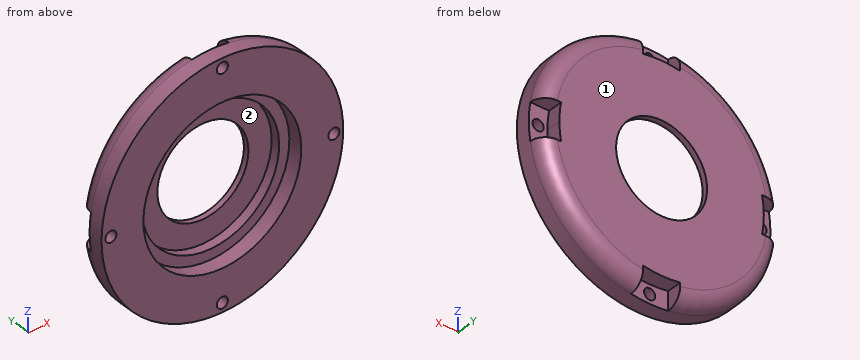
from build123d import *
from build123d.topology import SkipClean

# Parameters (mm, degrees)
SKETCH1_R           = 32.5
SKETCH1_R_2         = 27.5
BOSS_EXTRUDE1_DEPTH = 4
BOSS_EXTRUDE2_DEPTH = 4
SKETCH3_R           = 1.5
CUT_EXTRUDE1_DEPTH  = 6
BOSS_EXTRUDE4_START = -8
SKETCH7_R           = 25
BOSS_EXTRUDE4_DEPTH = 8
SKETCH8_R           = 27.5
SKETCH8_R_2         = 12.25
BOSS_EXTRUDE5_DEPTH = 4
SKETCH10_R          = 25
SKETCH10_R_2        = 12.25
BOSS_EXTRUDE6_DEPTH = 4
FILLET3_R           = 4
SKETCH11_R          = 21.25
CUT_EXTRUDE2_DEPTH  = 4
SKETCH14_R          = 18.5
CUT_EXTRUDE3_DEPTH  = 2.5


with BuildPart() as part:
    # Sketch1 → Boss-Extrude1 (new body)
    with BuildSketch(Plane(origin=(0, 0, 0), x_dir=(1, 0, 0), z_dir=(0, 1, 0))):
        with Locations(Location((0, 0, 0), (0, 0, 270))):
            Circle(SKETCH1_R)
        with Locations(Location((0, 0, 0), (0, 0, 270))):
            Circle(SKETCH1_R_2, mode=Mode.SUBTRACT)
    extrude(amount=BOSS_EXTRUDE1_DEPTH)

    # Sketch2 → Boss-Extrude2 (add)
    with SkipClean():  # the faces are left unmerged after this step: merging them gives an invalid solid
        with BuildSketch(Plane(origin=(0, 4, 0), x_dir=(1, 0, 0), z_dir=(0, 1, 0))):
            with BuildLine():
                ThreePointArc((-5, 32.113081447), (-22.980970389, 22.980970389), (-32.113081447, 5))
                Line((-32.113081447, 5), (-30, 5))
                Line((-30, 5), (-27.041634566, 5))
                ThreePointArc((-27.041634566, 5), (-19.445436483, 19.445436483), (-5, 27.041634566))
                Line((-5, 27.041634566), (-5, 32.113081447))
            make_face()
            with BuildLine():
                Line((-27.041634566, -5), (-32.113081447, -5))
                ThreePointArc((-32.113081447, -5), (-22.980970389, -22.980970389), (-5, -32.113081447))
                Line((-5, -32.113081447), (-5, -27.041634566))
                ThreePointArc((-5, -27.041634566), (-19.445436483, -19.445436483), (-27.041634566, -5))
            make_face()
            with BuildLine():
                Line((5, -27.041634566), (5, -32.113081447))
                ThreePointArc((5, -32.113081447), (22.980970389, -22.980970389), (32.113081447, -5))
                Line((32.113081447, -5), (27.041634566, -5))
                ThreePointArc((27.041634566, -5), (19.445436483, -19.445436483), (5, -27.041634566))
            make_face()
            with BuildLine():
                ThreePointArc((32.113081447, 5), (22.980970389, 22.980970389), (5, 32.113081447))
                Line((5, 32.113081447), (5, 27.041634566))
                ThreePointArc((5, 27.041634566), (19.445436483, 19.445436483), (27.041634566, 5))
                Line((27.041634566, 5), (32.113081447, 5))
            make_face()
        extrude(amount=BOSS_EXTRUDE2_DEPTH)

    # Sketch3 → Cut-Extrude1 (cut)
    with SkipClean():  # the faces are left unmerged after this step: merging them gives an invalid solid
        with BuildSketch(Plane(origin=(0, 4, 0), x_dir=(1, 0, 0), z_dir=(0, 1, 0))):
            with Locations(Location((0, 30, 0), (0, 0, 270))):
                Circle(SKETCH3_R)
            with Locations(Location((30, 0, 0), (0, 0, 270))):
                Circle(SKETCH3_R)
            with Locations(Location((0, -30, 0), (0, 0, 270))):
                Circle(SKETCH3_R)
            with Locations(Location((-30, 0, 0), (0, 0, 270))):
                Circle(SKETCH3_R)
        extrude(amount=-CUT_EXTRUDE1_DEPTH, mode=Mode.SUBTRACT)

    # Sketch7 → Boss-Extrude4 (add)
    # profile 1 of 5: a face of its own
    with BuildSketch(Plane(origin=(0, 8, 0), x_dir=(1, 0, 0), z_dir=(0, 1, 0)).offset(BOSS_EXTRUDE4_START)):
        with BuildLine():
            ThreePointArc((-27.041634566, 5), (-19.445436483, 19.445436483), (-5, 27.041634566))
            Line((-5, 27.041634566), (-5, 32.113081447))
            ThreePointArc((-5, 32.113081447), (-22.980970389, 22.980970389), (-32.113081447, 5))
            Line((-32.113081447, 5), (-27.041634566, 5))
        make_face()
    # profile 2 of 5: a face of its own
    with BuildSketch(Plane(origin=(0, 8, 0), x_dir=(1, 0, 0), z_dir=(0, 1, 0)).offset(BOSS_EXTRUDE4_START)):
        with BuildLine():
            Line((27.041634566, 5), (32.113081447, 5))
            ThreePointArc((32.113081447, 5), (22.980970389, 22.980970389), (5, 32.113081447))
            Line((5, 32.113081447), (5, 27.041634566))
            ThreePointArc((5, 27.041634566), (19.445436483, 19.445436483), (27.041634566, 5))
        make_face()
    # profile 3 of 5: a face of its own
    with BuildSketch(Plane(origin=(0, 8, 0), x_dir=(1, 0, 0), z_dir=(0, 1, 0)).offset(BOSS_EXTRUDE4_START)):
        with BuildLine():
            Line((5, -27.041634566), (5, -32.113081447))
            ThreePointArc((5, -32.113081447), (22.980970389, -22.980970389), (32.113081447, -5))
            Line((32.113081447, -5), (27.041634566, -5))
            ThreePointArc((27.041634566, -5), (19.445436483, -19.445436483), (5, -27.041634566))
        make_face()
    # profile 4 of 5: a face of its own
    with BuildSketch(Plane(origin=(0, 8, 0), x_dir=(1, 0, 0), z_dir=(0, 1, 0)).offset(BOSS_EXTRUDE4_START)):
        with BuildLine():
            Line((-27.041634566, -5), (-32.113081447, -5))
            ThreePointArc((-32.113081447, -5), (-22.980970389, -22.980970389), (-5, -32.113081447))
            Line((-5, -32.113081447), (-5, -27.041634566))
            ThreePointArc((-5, -27.041634566), (-19.445436483, -19.445436483), (-27.041634566, -5))
        make_face()
    # profile 5 of 5: a face of its own
    with BuildSketch(Plane(origin=(0, 8, 0), x_dir=(1, 0, 0), z_dir=(0, 1, 0)).offset(BOSS_EXTRUDE4_START)):
        with BuildLine():
            ThreePointArc((-27.041634566, -5), (-19.445436483, -19.445436483), (-5, -27.041634566))
            ThreePointArc((-5, -27.041634566), (0, -27.5), (5, -27.041634566))
            ThreePointArc((5, -27.041634566), (19.445436483, -19.445436483), (27.041634566, -5))
            ThreePointArc((27.041634566, -5), (27.385168893, -2.510482965), (27.5, 0))
            ThreePointArc((27.5, 0), (27.385168893, 2.510482965), (27.041634566, 5))
            ThreePointArc((27.041634566, 5), (19.445436483, 19.445436483), (5, 27.041634566))
            ThreePointArc((5, 27.041634566), (0, 27.5), (-5, 27.041634566))
            ThreePointArc((-5, 27.041634566), (-19.445436483, 19.445436483), (-27.041634566, 5))
            ThreePointArc((-27.041634566, 5), (-27.5, 0), (-27.041634566, -5))
        make_face()
        with Locations(Location((0, 0, 0), (0, 0, 270))):
            Circle(SKETCH7_R, mode=Mode.SUBTRACT)
    extrude(amount=BOSS_EXTRUDE4_DEPTH)

    # Sketch8 → Boss-Extrude5 (add)
    with BuildSketch(Plane(origin=(0, 0, 0), x_dir=(-1, 0, 0), z_dir=(0, -1, 0))):
        Circle(SKETCH8_R)
        with Locations(Location((0, 0, 0), (0, 0, 90))):
            Circle(SKETCH8_R_2, mode=Mode.SUBTRACT)
    extrude(amount=-BOSS_EXTRUDE5_DEPTH)

    # Sketch10 → Boss-Extrude6 (add)
    with BuildSketch(Plane(origin=(0, 4, 0), x_dir=(1, 0, 0), z_dir=(0, 1, 0))):
        Circle(SKETCH10_R)
        with Locations(Location((0, 0, 0), (0, 0, 90))):
            Circle(SKETCH10_R_2, mode=Mode.SUBTRACT)
    extrude(amount=BOSS_EXTRUDE6_DEPTH)

    # Fillet3
    fillet3_edges = [part.edges().sort_by_distance(p)[0] for p in [
        (22.980970389, 8, -22.980970389),
        (22.980970389, 8, 22.980970389),
        (-22.980970389, 8, 22.980970389),
        (-22.980970389, 8, -22.980970389),
    ]]
    fillet(fillet3_edges, radius=FILLET3_R - 0.0001)  # a hair under: the kernel refuses the full size

    # Sketch11 → Cut-Extrude2 (cut)
    with BuildSketch(Plane.XZ):
        with Locations(Location((0, 0, 0), (0, 0, 270))):
            Circle(SKETCH11_R)
    extrude(amount=-CUT_EXTRUDE2_DEPTH, mode=Mode.SUBTRACT)

    # Sketch14 → Cut-Extrude3 (cut)
    with BuildSketch(Plane.XZ.offset(-4)):
        with Locations(Location((0, 0, 0), (0, 0, 270))):
            Circle(SKETCH14_R)
    extrude(amount=-CUT_EXTRUDE3_DEPTH, mode=Mode.SUBTRACT)


solid = part.part
Input: part model. Units: mm. Frame: model coordinates. Face numbers are marked on the shaded views. Coordinates: 2 decimals unless noted, no trailing zeros. Loops run counter-clockwise (first coordinate to the right, second up) from the corner with the lowest first, then second, coordinate; pieces in that order, holes last.
(1) Material intervals for probe 1 along X at (y, z) = (3.2, 0); probe 2 along X at (y, z) = (1.1, -30); probe 3 along Z at (x, y) = (7, 3.75), sorted ascending.
(2) Pull-direction query (X, two-part tool) for the marked faces 1 and 2; classes: released by +X, released by -X, zero draft, split by the parting line, or undercut.
(3) Section A-A on x = 0. Return the cut outline in (y, z), then the cut area to 3 significant figures.
(4) Section C-C on y = 5.75. Return the cut outline in (x, z).
(5) First-contact query: pin 1 Ø13 at (x, z) = (0.5, -10) entering from -Y; pin 2 Ø22 at (x, z) = (0, 0) entering from +Y; pin 3 Ø1.6 at (x, z) = (-1, 30) entering from +Y; pin 4 Ø3 at (y, z) = (5, 28.5) entering from +X. Flat tips, straight axial feed; report the tip coordinate or a pass-through.
(6) Section B-B on y = 1.5. Return the cut outline in (x, z).
Data:
1. probe 1: x = -32.5 to -31.5, -28.5 to -21.25, 21.25 to 28.5, 31.5 to 32.5
1. probe 2: x = -12.5 to -1.5, 1.5 to 12.5
1. probe 3: z = -31.74 to -20.06, 20.06 to 31.74
2. face 1: zero draft
2. face 2: undercut
3. outline: (0, -32.5) - (4, -32.5) - (4, -31.5) - (0, -31.5) - close; (0, -28.5) - (4, -28.5) - (4, -27.5) - (8, -27.5) - (8, -12.25) - (6.5, -12.25) - (6.5, -18.5) - (4, -18.5) - (4, -21.25) - (0, -21.25) - close; (0, 21.25) - (4, 21.25) - (4, 18.5) - (6.5, 18.5) - (6.5, 12.25) - (8, 12.25) - (8, 27.5) - (4, 27.5) - (4, 28.5) - (0, 28.5) - close; (0, 31.5) - (4, 31.5) - (4, 32.5) - (0, 32.5) - close
3. area: 157 mm2
4. outline: (-31.71, -5) arc R32.1 ccw to (-5, -31.71) - (-5, -27.04) arc R27.5 ccw to (5, -27.04) - (5, -31.71) arc R32.1 ccw to (31.71, -5) - (27.04, -5) arc R27.5 ccw to (27.04, 5) - (31.71, 5) arc R32.1 ccw to (5, 31.71) - (5, 27.04) arc R27.5 ccw to (-5, 27.04) - (-5, 31.71) arc R32.1 ccw to (-31.71, 5) - (-27.04, 5) arc R27.5 ccw to (-27.04, -5) - close; hole circle Ø37 at (0, 0)
5. pin 1: stops at y = 6.5
5. pin 2: passes through
5. pin 3: stops at y = 4
5. pin 4: stops at x = 17.93
6. outline: circle Ø65 at (0, 0); hole circle Ø3 at (-30, 0); hole circle Ø42.5 at (0, 0); hole circle Ø3 at (0, -30); hole circle Ø3 at (0, 30); hole circle Ø3 at (30, 0)
